Here's how the part is built. I have some questions about the finished solid (model axes, mm). Coordinates: 2 decimals unless noted, no trailing zeros. Write each loop counter-clockwise with the first axis right and the second up, starting at its lowest first coordinate (ties: lowest second). Pieces come first, ordered by that corner, then holes. Notation, with made-up numbers: (67.25, 16.25) -> (123.25, 16.25) arc R15 ccw to (123.25, 45.25) -> close; hole circle Ø3 at (62.5, 55). An arc over 180 degrees is marked (long way). Use a Markdown table: item, result. Add a question column.
Item 1: Imagine slicing it at B-B, the plane z = 39.5. Write out the boundary of the cut face in (x, y).
Item 2: Imagine slicing it at A-A, the plane x = 26.5. Write out the boundary of the cut face in (y, z), and give its area (4 significant figures).
Item 3: Imagine slicing it at C-C, the plane x = 16. Write out the boundary of the cut face in (y, z).
Item 4: Imagine slicing it at D-D, the plane y = -2.05. Count the separate pieces of the cut face and the enclosed holes in it, and give its area (3 significant figures).
Item 5: If I drill on line 1 along Z through (x, y) = (0, -1.05); line 2 along Z through (x, y) = (42, -3.75); line 3 along Z through (x, y) = (25.5, -0.65), over which ranges is the centre line in solid material (lowest first)? Write a range as from..to.
Item 6: Will these pins go through, and if not, where does the flat tip stop? pin 1 Ø1.9 at (x, z) = (-17.42, -36.9) entering from -Y; pin 2 Ø3.5 at (x, z) = (-17.42, 153.2) entering from +Y; pin 3 Ø24.5 at (x, z) = (38, -18) entering from -Y.
Item 7: If we mould it in two halves opening along X, with no side actions, what happens to faces 1 (the flat face through (-22.423, -2, 57)), 2 (the flat face through (66.577, -2, 57)), 3 (the flat face through (28, -0.75, -30)), 4 (the flat face through (21, 0, 60))? For each: pulls with the +X half, pulls with the -X half, needs draft (parallel to the pull), parting line crosses it, or undercut.
```python
from build123d import *

# Parameters (mm, degrees)
F0_W     = 89
F0_H     = 200
F0_R     = 1.603513
F0_W_2   = 46.7
F0_H_2   = 27.2
F0_R_2   = 12
F1_DEPTH = 4
F2_R     = 3
F3_W     = 50.7
F3_H     = 30.8
F4_DEPTH = 3.25
F5_R     = 2.4


with BuildPart() as f1:
    # F0 (on Front) → F1 (new body)
    with BuildSketch(Plane.XZ):
        with Locations((22.076878, 58.203301)):
            Rectangle(F0_W, F0_H)
        with Locations((-17.421687, -36.900826)):
            Circle(F0_R, mode=Mode.SUBTRACT)
        with Locations((28.044092, -16.062529)):
            Rectangle(F0_W_2, F0_H_2, mode=Mode.SUBTRACT)
        with Locations((62.523074, -36.637016)):
            Circle(F0_R, mode=Mode.SUBTRACT)
        with Locations((42.562623, 35.063349)):
            Circle(F0_R_2, mode=Mode.SUBTRACT)
        with Locations((6.728478, 65.911161)):
            Circle(F0_R_2, mode=Mode.SUBTRACT)
        with Locations((-17.423122, 153.203301)):
            Circle(F0_R, mode=Mode.SUBTRACT)
        with Locations((6.728478, 128.332034)):
            Circle(F0_R_2, mode=Mode.SUBTRACT)
        with Locations((42.562623, 97.028293)):
            Circle(F0_R_2, mode=Mode.SUBTRACT)
        with Locations((62.576878, 153.203301)):
            Circle(F0_R, mode=Mode.SUBTRACT)
    extrude(amount=F1_DEPTH)

    # F2
    f2_edges = [f1.edges().sort_by_distance(p)[0] for p in [
        (-22.423122, -2, 158.203301),
        (66.576878, -2, 158.203301),
        (66.576878, -2, -41.796699),
        (-22.423122, -2, -41.796699),
    ]]
    fillet(f2_edges, radius=F2_R)

    # F3 (on face) → F4 (cut)
    with BuildSketch(Plane.XZ.offset(4)):
        with Locations((28.044092, -16.062529)):
            Rectangle(F3_W, F3_H)
    extrude(amount=-F4_DEPTH, mode=Mode.SUBTRACT)

    # F5
    f5_edges = [f1.edges().sort_by_distance(p)[0] for p in [
        (2.694092, -2.375, -0.662529),
        (53.394092, -2.375, -31.462529),
        (2.694092, -2.375, -31.462529),
        (53.394092, -2.375, -0.662529),
    ]]
    fillet(f5_edges, radius=F5_R)


solid = f1.part
```
Ans:
| question | item | result |
|---|---|---|
| 1 | outline | (-22.42, -4) -> (31.41, -4) -> (31.41, 0) -> (-22.42, 0) -> close; (53.71, -4) -> (66.58, -4) -> (66.58, 0) -> (53.71, 0) -> close |
| 2 | outline | (-4, -41.8) -> (0, -41.8) -> (0, -29.66) -> (-0.75, -29.66) -> (-0.75, -31.46) -> (-4, -31.46) -> close; (-4, -0.66) -> (-0.75, -0.66) -> (-0.75, -2.46) -> (0, -2.46) -> (0, 158.2) -> (-4, 158.2) -> close |
| 2 | area | 679.5 mm^2 |
| 3 | outline | (-4, -41.8) -> (0, -41.8) -> (0, -29.66) -> (-0.75, -29.66) -> (-0.75, -31.46) -> (-4, -31.46) -> close; (-4, -0.66) -> (-0.75, -0.66) -> (-0.75, -2.46) -> (0, -2.46) -> (0, 58.29) -> (-4, 58.29) -> close; (-4, 73.53) -> (0, 73.53) -> (0, 120.71) -> (-4, 120.71) -> close; (-4, 135.95) -> (0, 135.95) -> (0, 158.2) -> (-4, 158.2) -> close |
| 4 | separate pieces | 1 |
| 4 | enclosed holes | 9 |
| 4 | area | 14,400 mm^2 |
| 5 | line 1 | z = -41.8..55.97, 75.85..118.4, 138.27..158.2 |
| 5 | line 2 | z = -41.8..-31.46, -0.66..23.08, 47.05..85.04, 109.02..158.2 |
| 5 | line 3 | z = -41.8..-29.66, -2.46..158.2 |
| 6 | pin 1 | passes through |
| 6 | pin 2 | stops at y = 0 |
| 6 | pin 3 | stops at y = -0.75 |
| 7 | face 1 | pulls with the -X half |
| 7 | face 2 | pulls with the +X half |
| 7 | face 3 | undercut |
| 7 | face 4 | needs draft |
